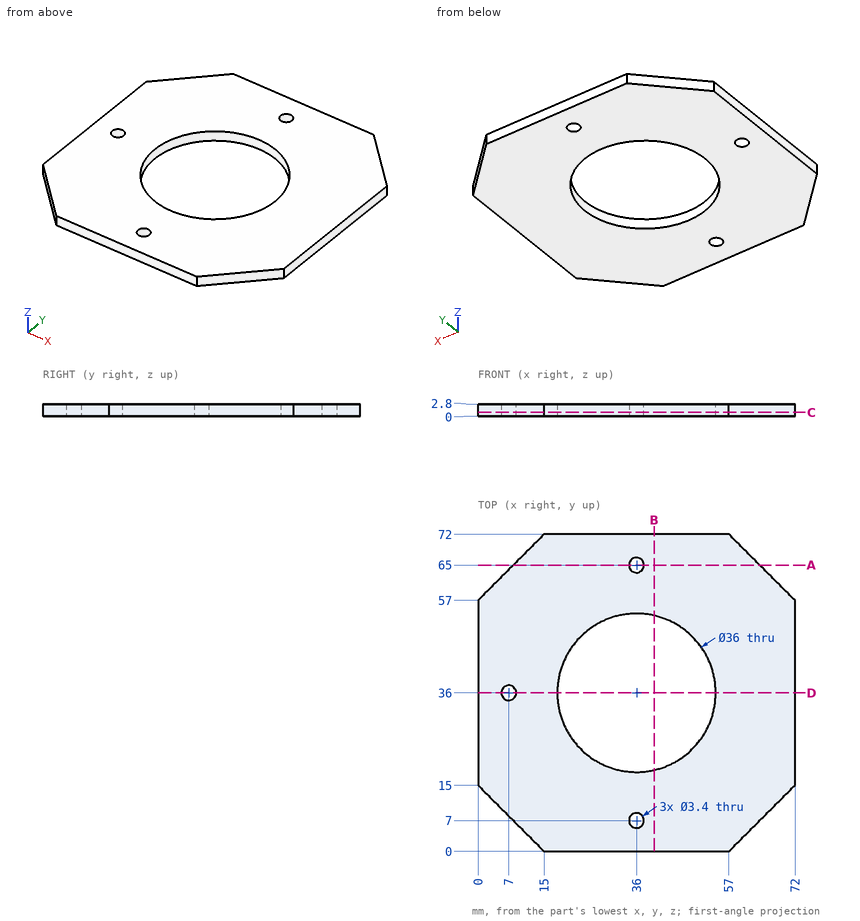
The drawing under review shows one solid part. Ordinate dimensions are in mm from its lowest x, y, z. Round coordinates to 2 decimals unless told otherwise and drop trailing zeros. Loops run counter-clockwise (first coordinate to the right, second up) from the corner with the lowest first, then second, coordinate; pieces in that order, holes last. Notation, with made-up numbers: (26, -8) - (50, -8) arc R13 ccw to (50, -3) - close; hole circle Ø4 at (89.25, 51.5). An arc over 180 degrees is marked (long way). One line per item, written item: value. Start each with the question number.
1) Insertion check: pin 1 Ø5.5 at (x, y) = (7, 36) entering from -Z; pin 2 Ø1 at (x, z) = (63.5, 1.5) entering from +Y. Each pin has a flat end and moves straight along its axis. Give the tip position at first contact, or say it passes through.
2) Consider section A-A on y = 65. Give the boundary of the cut face in (x, z).
3) Consider section D-D on y = 36. Give the boundary of the cut face in (x, z).
4) Consider section B-B on x = 40. Give the boundary of the cut face in (y, z), then the cut area to 3 significant figures.
5) To check wall thickness, follow L1, parallel to Y at x = 36, z = 2.65; L2, parallel to X at y = 35, z = 0.35; L3, parallel to X at y = 6, z = 0.65. State the ranges of each line that lie inside material, in increasing order. Write a range as from..to.
6) Consider section C-C on z = 0.9. Give the boundary of the cut face in (x, y).
Reported:
1. pin 1: stops at z = 0
1. pin 2: stops at y = 66
2. outline: (8, 0) - (34.3, 0) - (34.3, 2.8) - (8, 2.8) - close; (37.7, 0) - (64, 0) - (64, 2.8) - (37.7, 2.8) - close
3. outline: (0, 0) - (5.3, 0) - (5.3, 2.8) - (0, 2.8) - close; (8.7, 0) - (18, 0) - (18, 2.8) - (8.7, 2.8) - close; (54, 0) - (72, 0) - (72, 2.8) - (54, 2.8) - close
4. outline: (0, 0) - (18.45, 0) - (18.45, 2.8) - (0, 2.8) - close; (53.55, 0) - (72, 0) - (72, 2.8) - (53.55, 2.8) - close
4. area: 103 mm^2
5. L1: y = 0..5.3, 8.7..18, 54..63.3, 66.7..72
5. L2: x = 0..5.63, 8.37..18.03, 53.97..72
5. L3: x = 9..34.63, 37.37..63
6. outline: (0, 15) - (15, 0) - (57, 0) - (72, 15) - (72, 57) - (57, 72) - (15, 72) - (0, 57) - close; hole circle Ø3.4 at (7, 36); hole circle Ø36 at (36, 36); hole circle Ø3.4 at (36, 7); hole circle Ø3.4 at (36, 65)
